```python
from build123d import *

# Parameters (mm, degrees)
F1_DEPTH = 8
F3_R     = 3
F2_R     = 2.5
F4_DEPTH = 4.572962


with BuildPart() as f1:
    # F0 (on Top) → F1 (new body)
    with BuildSketch(Plane.XY):
        Polygon((0, 0), (0, 15.2), (-2, 15.2), (-2, -0.986916), (13, -0.986916), (13, 5.2), (2.571962, 5.2), (2.571962, 15.2), (0.571962, 15.2), (0.538318, 15.2), (0.538318, 3.2), (11, 3.2), (11, 0), align=None)
    extrude(amount=-F1_DEPTH)

    # F3
    f3_edges = [f1.edges().sort_by_distance(p)[0] for p in [
        (1.55514, 15.2, 0),
        (-1, 15.2, 0),
        (-1, 15.2, -8),
        (1.55514, 15.2, -8),
    ]]
    fillet(f3_edges, radius=F3_R)

    # F2 (on face) → F4 (cut, through all)
    with BuildSketch(Plane.YZ.offset(2.571962)):
        with Locations((10.2, -4)):
            Circle(F2_R)
    extrude(amount=-F4_DEPTH, mode=Mode.SUBTRACT)


solid = f1.part
```
Can you work these out from the model? Positions are in its coordinate system, mm. A direction names the side the tool comes from. Give positions to 0.01 mm unless a question says otherwise; leave off trailing zeros. Write each loop counter-clockwise with the first axis right and the second up, starting at its lowest first coordinate (ties: lowest second). Pieces come first, ordered by that corner, then holes. Notation, with made-up numbers: (-12.75, -23) -> (23.25, -23) arc R12 cw to (23.25, 0) -> close; hole circle Ø3 at (0, 1). An arc over 180 degrees is marked (long way). One line per item, written item: value.
Q1. Which directions (+Z, -Z, +X, -X, +Y, -Y) give clear straight access to the entire face, cutting with the end or side of a thin tool? Please do faces 1 (the face through (2, 15.2, -4)), 2 (the face through (8, 5.2, -4)), 3 (the face through (0.538, 8, -2)), 4 (the face through (4, 4, 0)), 5 (the face through (6, 0, -4)).
Results found:
face 1: +Z, -Z, +X, -X, +Y
face 2: +Z, -Z, +X, +Y
face 3: +Z, -Z, +Y
face 4: +Z, +X, -X, +Y, -Y
face 5: +Z, -Z
Q2. Imagine slicing it at D-D on x = 9.25. Please give me the cut outline in (y, z).
Results found:
outline: (-0.99, -8) -> (0, -8) -> (0, 0) -> (-0.99, 0) -> close; (3.2, -8) -> (5.2, -8) -> (5.2, 0) -> (3.2, 0) -> close
Q3. Imagine slicing it at A-A on y = 7. Please give me the cut outline in (x, z), and give its area (3 significant figures).
Results found:
outline: (-2, -8) -> (0, -8) -> (0, 0) -> (-2, 0) -> close; (0.54, -8) -> (2.57, -8) -> (2.57, 0) -> (0.54, 0) -> close
area: 32.3 mm^2
Q4. Imagine slicing it at B-B on z = -4. Please give me the cut outline in (x, y), and give its area (3 significant figures).
Results found:
outline: (-2, -0.99) -> (13, -0.99) -> (13, 5.2) -> (2.57, 5.2) -> (2.57, 7.7) -> (0.54, 7.7) -> (0.54, 3.2) -> (11, 3.2) -> (11, 0) -> (0, 0) -> (0, 7.7) -> (-2, 7.7) -> close; (-2, 12.7) -> (0, 12.7) -> (0, 15.2) -> (-2, 15.2) -> close; (0.54, 12.7) -> (2.57, 12.7) -> (2.57, 15.2) -> (0.54, 15.2) -> close
area: 76.7 mm^2
Q5. Imagine slicing it at C-C on x = -1. Please give me the cut outline in (y, z), and give its area (3 significant figures).
Results found:
outline: (-0.99, -8) -> (12.2, -8) arc R3 ccw to (15.2, -5) -> (15.2, -3) arc R3 ccw to (12.2, 0) -> (-0.99, 0) -> close; hole circle Ø5 at (10.2, -4)
area: 106 mm^2
Q6. We'd pull the mould along X, two halves only. Please class faces 6 (the face through (0, 7, -4)), 7 (the face through (4, 4, -8)), 8 (the face through (-2, 7, -4)): +X half, -X half, draft (parallel to the pull), parting line (faces both ways), or undercut.
Results found:
face 6: undercut
face 7: draft
face 8: -X half
Q7. Please list where these lines run through material, in increasing order: line 1 (X direction, y = 7, z = -4.5); line 2 (Z direction, x = 1.05, y = 10.2); line 3 (Y direction, x = 4, z = -5.5). Write a range as [from, to].
Results found:
line 1: x = [-2, 0], [0.54, 2.57]
line 2: z = [-8, -6.5], [-1.5, 0]
line 3: y = [-0.99, 0], [3.2, 5.2]
Q8. For P1, Ø1, axis at y = 12.5, z = -3.5, coming from the +X side; P2, Ø4, axis at x = 7, z = -4.5, coming from the +Y side, each with a flat end and sliding along its axis, tell me the tip position at first contact or that it passes through.
Results found:
P1: stops at x = 2.57
P2: stops at y = 5.2
